Here's the drawing with two shaded views (mm, measured from the low corner). I have some questions. Give positions to 0.01 mm unless a question says otherwise; leave off trailing zeros. Loops run counter-clockwise (first coordinate to the right, second up) from the corner with the lowest first, then second, coordinate; pieces in that order, holes last. Notation, with made-up numbers: M 65.5,85 L 88.5,85 A30 cw 88.5,114 Z; hole C -5,5.5 d10. An arc over 180 degrees is marked long. Write item = value, one per line. Start each with the question number.
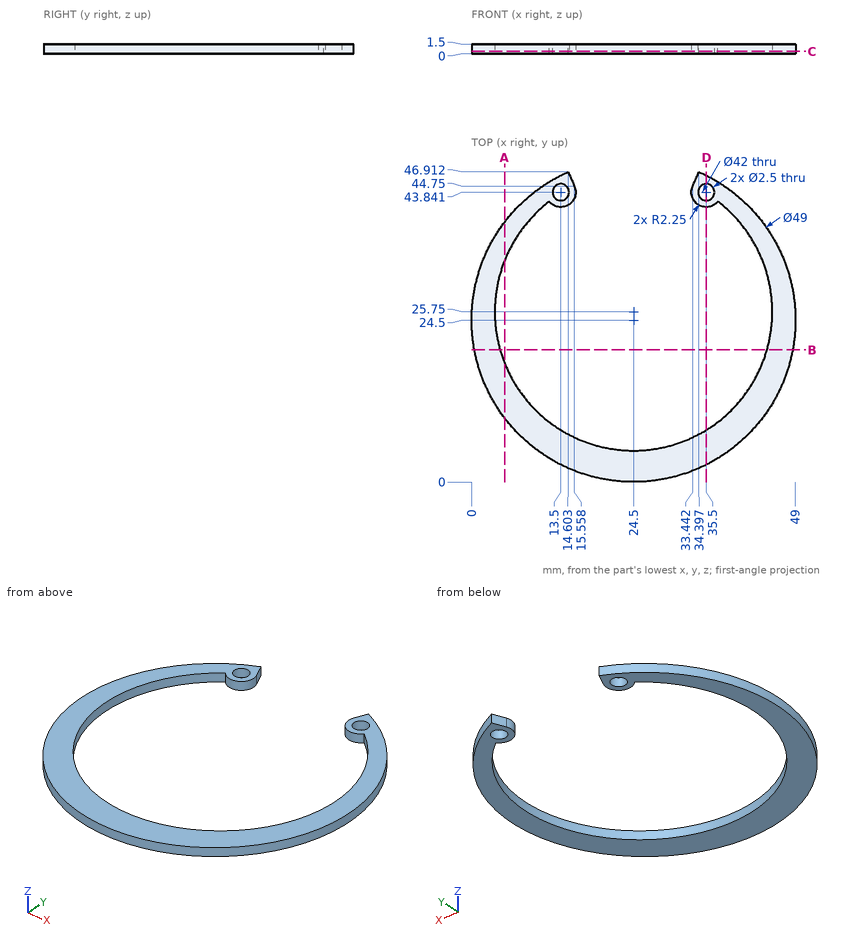
Q1. If we section it at A-A, the plane x = 5: List the corners of the cut face in (y, z) for me (1 decimal), then the cut area to 3 significant figures.
Q2. If I drill on line 1 along Y through (x, z) = (35.5, 0.9); line 2 along X through (y, z) = (26, 1.3) (1 decimal); line 3 along X through (y, z) = (39, 0.3), over which ranges is the centre line in solid material (lowest first)?
Q3. If we section it at C-C, the plane z = 0.4: State how many separate pieces and enclosed holes the cut face has, then the cut area to 3 significant figures.
Q4. Will these pins go through, and if not, where does the flat tip stop? pin 1 (3 mm diameter, centred on x = 13.5, y = 43.84, fed in from -Z); pin 2 (2 mm diameter, centred on x = 35.5, y = 43.84, fed in from -Z).
Q5. If we section it at D-D, the plane x = 35.5: List the corners of the cut face in (y, z) for me.
Q6. If we section it at B-B, the plane y = 20: List the corners of the cut face in (x, z) for me.
Resolved:
q1.outline = M 9.7,0 L 18,0 L 18,1.5 L 9.7,1.5 Z; M 33.5,0 L 39.3,0 L 39.3,1.5 L 33.5,1.5 Z
q1.area = 21.1 mm²
q2.line_1 = 2.61 to 7.86, 41.59 to 42.59, 45.09 to 46.39
q2.line_2 = 0 to 3.5, 45.5 to 49
q2.line_3 = 4.75 to 8.21, 40.79 to 44.25
q3.separate_pieces = 1
q3.enclosed_holes = 2
q3.area = 460 mm²
q4.pin_1 = 0
q4.pin_2 = through
q5.outline = M 2.61,0 L 7.86,0 L 7.86,1.5 L 2.61,1.5 Z; M 41.59,0 L 42.59,0 L 42.59,1.5 L 41.59,1.5 Z; M 45.09,0 L 46.39,0 L 46.39,1.5 L 45.09,1.5 Z
q6.outline = M 0.42,0 L 4.3,0 L 4.3,1.5 L 0.42,1.5 Z; M 44.7,0 L 48.58,0 L 48.58,1.5 L 44.7,1.5 Z
